CAD build for the part. Positions are in the model's coordinates, mm. Face numbers are marked on the shaded views. A direction names the side the tool comes from. Give positions to 0.01 mm unless a question says otherwise; leave off trailing zeros. Order: outer loops, then holes, each group sorted by start corner. A loop starts at its lowest first (then second) coordinate and runs counter-clockwise, first axis right, second up. Notation, with made-up numbers: (32, 16) -> (88, 16) arc R26 ccw to (88, 52) -> close; hole circle Ø8 at (-14, 11). An arc over 180 degrees is marked (long way). Use one line per item in the form item = value. Start each with the question number.
1) Cut at B-B, the plane x = 6. Give the cut face in (y, z) (3 decimals), and give its area (3 significant figures).
2) Cut at C-C, the plane z = 0. Give the cut face in (x, y) (3 decimals).
3) Probe line 1 (Y direction, x = 2.25, z = -7.5) (3 decimals); line 2 (X direction, y = -2.75, z = -6.75); line 3 (X direction, y = -8.25, z = -9.25) (3 decimals). List the from-to ranges inside material, lowest first.
4) Cut at D-D, the plane y = -11.5. Give the cut face in (x, z) (3 decimals).
5) Mould opens along X. For the marked faces 4, 5 and 6 say: pulls with the +X half, pulls with the -X half, needs draft (parallel to the pull), parting line crosses it, or undercut.
6) Drop flat-ended pins along their axis: P1, Ø3, axis at y = -8.5, z = 0, coming from the +X side; P2, Ø5.5, axis at x = 2.5, z = 5, coming from the -Y side; P3, Ø3, axis at y = -8.89, z = -8.128, coming from the +X side (3 decimals). Give the stop position or say it passes through.
7) Cut at A-A, the plane y = -8.89. Give the cut face in (x, z) (3 decimals), and give its area (3 significant figures).
8) Tool access for the marked faces 1, 2 and 3: list every direction of +Z, -Z, +X, -X, +Y, -Y with a clear straight run to the whole face (end or side of a thin tool).
from build123d import *

# Parameters (mm, degrees)
SKETCH1_W             = 20.32
SKETCH1_H             = 22.86
BOSS_EXTRUDE1_DEPTH   = 3.175
FILLET1_R             = 2.54
FILLET2_R             = 2.54
CUT_EXTRUDE2_DEPTH    = 4.175
FILLET3_R             = 2.54
FILLET4_R             = 2.54
SKETCH4_W             = 3.175
SKETCH4_H             = 22.86
BOSS_EXTRUDE2_DEPTH   = 12.7
FILLET6_R             = 5.08
SKETCH5_R             = 12.7
CUT_EXTRUDE4_DEPTH    = 13.7
F_4_40_TAPPED_HOLE3_D = 2.2606
CUT_EXTRUDE6_DEPTH    = 16.8750001


with BuildPart() as part:
    # Sketch1 → Boss-Extrude1 (new body)
    with BuildSketch(Plane(origin=(0, 0, 0), x_dir=(1, 0, 0), z_dir=(0, 1, 0))):
        Rectangle(SKETCH1_W, SKETCH1_H)
    extrude(amount=BOSS_EXTRUDE1_DEPTH)

    # Fillet1
    fillet1_edges = [part.edges().sort_by_distance(p)[0] for p in [
        (10.16, 1.5875, -11.43),
    ]]
    fillet(fillet1_edges, radius=FILLET1_R)

    # Fillet2
    fillet2_edges = [part.edges().sort_by_distance(p)[0] for p in [
        (10.16, 1.5875, 11.43),
    ]]
    fillet(fillet2_edges, radius=FILLET2_R)

    # Sketch2 → Cut-Extrude2 (cut, through all)
    with BuildSketch(Plane.XZ):
        with BuildLine():
            Line((5.08, -5.08), (10.16, -5.08))
            Line((10.16, -5.08), (10.16, 5.08))
            Line((10.16, 5.08), (5.08, 5.08))
            ThreePointArc((5.08, 5.08), (0, 0), (5.08, -5.08))
        make_face()
    extrude(amount=-CUT_EXTRUDE2_DEPTH, mode=Mode.SUBTRACT)

    # Fillet3
    fillet3_edges = [part.edges().sort_by_distance(p)[0] for p in [
        (10.16, 1.5875, 5.08),
    ]]
    fillet(fillet3_edges, radius=FILLET3_R)

    # Fillet4
    fillet4_edges = [part.edges().sort_by_distance(p)[0] for p in [
        (10.16, 1.5875, -5.08),
    ]]
    fillet(fillet4_edges, radius=FILLET4_R)

    # Sketch4 → Boss-Extrude2 (add)
    with BuildSketch(Plane.XZ):
        with Locations((-8.5725, 0)):
            Rectangle(SKETCH4_W, SKETCH4_H)
    extrude(amount=BOSS_EXTRUDE2_DEPTH)

    # Fillet6
    fillet6_edges = [part.edges().sort_by_distance(p)[0] for p in [
        (-6.985, 0, 0),
    ]]
    fillet(fillet6_edges, radius=FILLET6_R)

    # Sketch5 → Cut-Extrude4 (cut, through all)
    with BuildSketch(Plane.XZ):
        with Locations((5.08, 0)):
            Circle(SKETCH5_R)
    extrude(amount=CUT_EXTRUDE4_DEPTH, mode=Mode.SUBTRACT)

    # #4-40 Tapped Hole3 (through all)
    with Locations(Plane(origin=(-6.985, 0, 0), x_dir=(0, 0, -1), z_dir=(1, 0, 0))):
        with Locations((-8.128, -8.89), (8.128, -8.89)):
            Hole(F_4_40_TAPPED_HOLE3_D / 2)

    # Sketch11 → Cut-Extrude6 (cut, through all)
    with BuildSketch(Plane(origin=(0, 3.175, 0), x_dir=(1, 0, 0), z_dir=(0, 1, 0))):
        with BuildLine():
            Line((6.985, 9.8298), (4.445, 9.8298))
            ThreePointArc((4.445, 9.8298), (2.7432, 8.128), (4.445, 6.4262))
            Line((4.445, 6.4262), (6.985, 6.4262))
            ThreePointArc((6.985, 6.4262), (8.6868, 8.128), (6.985, 9.8298))
        make_face()
        with BuildLine():
            Line((4.445, -6.4262), (6.985, -6.4262))
            ThreePointArc((6.985, -6.4262), (8.6868, -8.128), (6.985, -9.8298))
            Line((6.985, -9.8298), (4.445, -9.8298))
            ThreePointArc((4.445, -9.8298), (2.7432, -8.128), (4.445, -6.4262))
        make_face()
    extrude(amount=-CUT_EXTRUDE6_DEPTH, mode=Mode.SUBTRACT)


solid = part.part
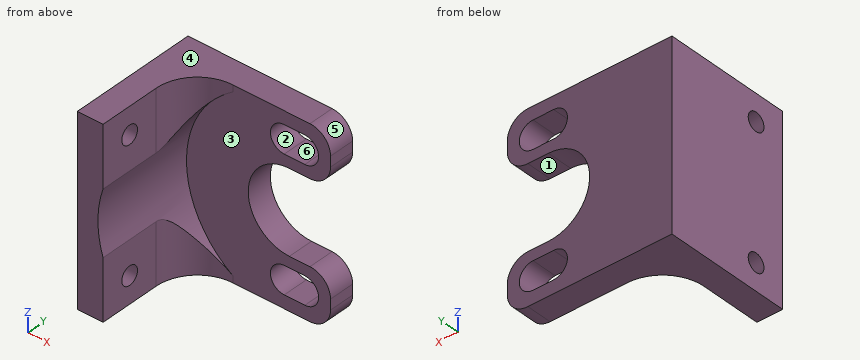
Result:
q1.outline = (0, -11.43) -> (3.175, -11.43) -> (3.175, -9.83) -> (0, -9.83) -> close; (0, -6.426) -> (3.175, -6.426) -> (3.175, -5.08) -> (0, -5.08) -> close; (0, 5.08) -> (3.175, 5.08) -> (3.175, 6.426) -> (0, 6.426) -> close; (0, 9.83) -> (3.175, 9.83) -> (3.175, 11.43) -> (0, 11.43) -> close
q1.area = 18.7 mm²
q2.outline = (-10.16, -12.7) -> (-7.62, -12.7) -> (-7.62, 0) -> (0, 0) -> (0, 3.175) -> (-10.16, 3.175) -> close
q3.line_1 = 0 to 3.175
q3.line_2 = -10.16 to -6.42
q3.line_3 = -10.16 to -6.985
q4.outline = (-10.16, -11.43) -> (-6.985, -11.43) -> (-6.985, -3.966) arc R12.7 cw to (-6.985, 3.966) -> (-6.985, 11.43) -> (-10.16, 11.43) -> close
q5.face_4 = needs draft
q5.face_5 = pulls with the +X half
q5.face_6 = undercut
q6.P1 = -7.53
q6.P2 = 0
q6.P3 = -6.985
q7.outline = (-10.16, -11.43) -> (-6.985, -11.43) -> (-6.985, -9.258) -> (-10.16, -9.258) -> close; (-10.16, -6.998) -> (-6.985, -6.998) -> (-6.985, -3.966) arc R12.7 cw to (-6.985, 3.966) -> (-6.985, 6.998) -> (-10.16, 6.998) -> close; (-10.16, 9.258) -> (-6.985, 9.258) -> (-6.985, 11.43) -> (-10.16, 11.43) -> close
q7.area = 54.9 mm²
q8.face_1 = +X, +Y, -Y
q8.face_2 = +Y, -Y
q8.face_3 = +X, -Y
